Geometry: final body of the model. Coordinates: model frame, mm. A direction names the side the tool comes from. Coordinates: 2 decimals unless noted, no trailing zeros. Order: outer loops, then holes, each group sorted by start corner. A loop starts at its lowest first (then second) coordinate and runs counter-clockwise, first axis right, second up. Notation, with made-up numbers: (15, 36) -> (21, 36) arc R23 cw to (21, 51) -> close; hole circle Ø2 at (-28, 74.5). An arc over 180 degrees is marked (long way). Answer in a Markdown table with one row per item. Add a question column.
1) Contact query for flat-ended pins moving along their axis: P1, Ø10, axis at x = -7.5, y = 27, coming from the -Z side; P2, Ø2, axis at x = -24, z = 77.5, coming from the +Y side; P3, Ø1, axis at y = 39.5, z = 77, coming from the -X side. Output: stop coordinate, or through.
2) Section query B-B on x = -39. Return the cut outline in (y, z).
3) Pull-direction query (Y, two-part tool) for faces 5 (the face through (-0.99, 46.9, 70.99)), 6 (the face through (-28, 2, 37)), 7 (the face through (-2, 64, 69)), 8 (the face through (-28, 0, 38)); classes: +Y half, -Y half, draft (parallel to the pull), parting line (faces both ways), or undercut.
4) Ray query, line 1 (X direction, y = 50, z = 71); line 2 (Z direction, x = -24, y = 7.5); line 3 (Y direction, x = -32, z = 65). Return the intervals inside material, ascending. Write a range as from..to.
5) Section query A-A on z = 27. Return the cut outline in (x, y), then the cut area to 3 significant figures.
6) Section query D-D on z = 47. Return the cut outline in (x, y).
7) Section query C-C on y = 46. Return the cut outline in (x, z), then the cut area to 3 significant figures.
8) Set-up query: faces 1 (the face through (0, 29, 68)), 2 (the face through (-1, 5, 15)), 3 (the face through (-9, 34, 76)), 4 (the face through (-10, 52, 77)). Return all of +Z, -Z, +X, -X, +Y, -Y with unobstructed straight access to the full face (end or side cutting, diameter ignored); none if empty.
```python
from build123d import *

# Parameters (mm, degrees)
EXTRUDE_1_DEPTH     = 76
CUT_EXTRUDE_1_DEPTH = 70
EXTRUDE_2_DEPTH     = 2


with BuildPart() as part:
    # 草图1 → 凸台-拉伸1 (new body)
    with BuildSketch(Plane.XY):
        Polygon((-55.5, 0), (0, 0), (0, 92), (-2, 92), (-2, 2), (-55.5, 2), align=None)
    extrude(amount=EXTRUDE_1_DEPTH)

    # 草图2 → 切除-拉伸1 (cut)
    with BuildSketch(Plane(origin=(0, 0, 0), x_dir=(0, 0, -1), z_dir=(1, 0, 0))):
        with BuildLine():
            Line((-30, 5), (0, 5))
            Line((0, 5), (0, 87))
            Line((0, 87), (-30, 87))
            ThreePointArc((-30, 87), (-71, 46), (-30, 5))
        make_face()
    extrude(amount=-CUT_EXTRUDE_1_DEPTH, mode=Mode.SUBTRACT)

    # 草图3 → 凸台-拉伸2 (add)
    with BuildSketch(Plane.XY.offset(76)):
        Polygon((0, 92), (-10, 92), (-10, 10), (-55.5, 10), (-55.5, 0), (0, 0), align=None)
    extrude(amount=EXTRUDE_2_DEPTH)


solid = part.part
```
Result:
| question | item | result |
|---|---|---|
| 1 | P1 | z = 76 |
| 1 | P2 | y = 10 |
| 1 | P3 | x = -10 |
| 2 | outline | (0, 0) -> (2, 0) -> (2, 76) -> (10, 76) -> (10, 78) -> (0, 78) -> close |
| 3 | face 5 | undercut |
| 3 | face 6 | +Y half |
| 3 | face 7 | draft |
| 3 | face 8 | -Y half |
| 4 | line 1 | -2..0 |
| 4 | line 2 | 76..78 |
| 4 | line 3 | 0..2 |
| 5 | outline | (-55.5, 0) -> (0, 0) -> (0, 5) -> (-2, 5) -> (-2, 2) -> (-55.5, 2) -> close; (-2, 87) -> (0, 87) -> (0, 92) -> (-2, 92) -> close |
| 5 | area | 127 mm2 |
| 6 | outline | (-55.5, 0) -> (0, 0) -> (0, 8.69) -> (-2, 8.69) -> (-2, 2) -> (-55.5, 2) -> close; (-2, 83.31) -> (0, 83.31) -> (0, 92) -> (-2, 92) -> close |
| 7 | outline | (-10, 76) -> (-2, 76) -> (-2, 71) -> (0, 71) -> (0, 78) -> (-10, 78) -> close |
| 7 | area | 30.0 mm2 |
| 8 | face 1 | +Z, -Z, +X, +Y, -Y |
| 8 | face 2 | -Z, +X, -X |
| 8 | face 3 | -Z, -X, +Y |
| 8 | face 4 | +Z, -Z, -X, +Y |
